Here's how the part is built. I have some questions about the finished solid (model axes, mm). A direction names the side the tool comes from. Coordinates: 2 decimals unless noted, no trailing zeros. Write each loop counter-clockwise with the first axis right and the second up, starting at its lowest first coordinate (ties: lowest second). Pieces come first, ordered by that corner, then holes. Notation, with made-up numbers: (26.5, 31.5) -> (53.5, 31.5) arc R26 cw to (53.5, 48.5) -> close; hole circle Ø11 at (78, 75). An arc over 180 degrees is marked (long way). Use CSV: the item, a comma, the result in double quotes. Start each with the question number.
```python
from build123d import *

# Parameters (mm, degrees)
SKETCH1_R           = 6.35
SKETCH1_R_2         = 1.8288
BOSS_EXTRUDE1_DEPTH = 6.35
SKETCH2_W           = 26.667
SKETCH2_H           = 26.667
BOSS_EXTRUDE2_DEPTH = 6.35


with BuildPart() as part:
    # Sketch1 → Boss-Extrude1 (new body)
    with BuildSketch(Plane(origin=(0, 0, 0), x_dir=(1, 0, 0), z_dir=(0, 1, 0))):
        Polygon((-35.064474094, 47.36223941), (-35.064474094, 7.36323941), (-35.064474094, -30.73676059), (3.035525906, -30.73676059), (3.035525906, 7.36323941), (3.035525906, 47.36223941), align=None)
        with Locations(Location((-16.014474094, -11.68676059, 0), (0, 0, 270))):
            Circle(SKETCH1_R, mode=Mode.SUBTRACT)
        with Locations(Location((-16.014474094, -21.46576059, 0), (0, 0, 270))):
            Circle(SKETCH1_R_2, mode=Mode.SUBTRACT)
        with Locations(Location((-22.929271308, -18.601557803, 0), (0, 0, 270))):
            Circle(SKETCH1_R_2, mode=Mode.SUBTRACT)
        with Locations(Location((-25.793474094, -11.68676059, 0), (0, 0, 270))):
            Circle(SKETCH1_R_2, mode=Mode.SUBTRACT)
        with Locations(Location((-22.929271308, -4.771963377, 0), (0, 0, 270))):
            Circle(SKETCH1_R_2, mode=Mode.SUBTRACT)
        with Locations(Location((-16.014474094, -1.90776059, 0), (0, 0, 270))):
            Circle(SKETCH1_R_2, mode=Mode.SUBTRACT)
        with Locations(Location((-9.099676881, -4.771963377, 0), (0, 0, 270))):
            Circle(SKETCH1_R_2, mode=Mode.SUBTRACT)
        with Locations(Location((-6.235474094, -11.68676059, 0), (0, 0, 270))):
            Circle(SKETCH1_R_2, mode=Mode.SUBTRACT)
        with Locations(Location((-9.099676881, -18.601557803, 0), (0, 0, 270))):
            Circle(SKETCH1_R_2, mode=Mode.SUBTRACT)
    extrude(amount=BOSS_EXTRUDE1_DEPTH)

    # Sketch2 → Boss-Extrude2 (add)
    with BuildSketch(Plane(origin=(0, 6.35, 0), x_dir=(1, 0, 0), z_dir=(0, 1, 0))):
        with Locations((-16.014474094, 47.36223941)):
            Rectangle(SKETCH2_W, SKETCH2_H)
    extrude(amount=-BOSS_EXTRUDE2_DEPTH)


solid = part.part
```
Item 1: Which directions (+Z, -Z, +X, -X, +Y, -Y) give clear straight access to the entire face, cutting with the end or side of a thin tool? Please do faces 5 (the cylindrical face through (-27.58, 3.13, 11.29)), 6 (the flat face through (0, 3, -47.362)), 7 (the flat face through (-29.348, 3, -54)).
Item 2: Thinking about a two-plate mould opening in Z: for faces 1 (the cylindrical face through (-21.116, 3.131, 4.534)), 2 (the flat face through (-16, 0, -16)), 3 (the flat face through (-32, 3, -47.362)), 4 (the cylindrical face through (-15.47, 3.13, 23.21)), which applies, +Z half, -Z half, draft (parallel to the pull), parting line (faces both ways), or undercut?
Item 3: I'm going to push flat-ended pins straight in: pin 1 (3 mm diameter, centred on x = -31.5, y = 2, fed in from -Z); pin 2 (3.5 mm diameter, centred on x = -9.1, z = 4.77, fed in from +Y); pin 3 (2 mm diameter, centred on y = 5, z = -49, fed in from +X); pin 4 (1.9 mm diameter, centred on y = 4.5, z = -57, fed in from -X). Where does each tip first touch, or does it pass through?
Item 4: If I drill on line 1 along Z through (x, y) = (-7.5, 4); line 2 along Z through (x, y) = (-31.5, 3.25); line 3 along X through (y, z) = (3, -47.5), over which ranges is the centre line in solid material (lowest first)?
Item 5: I want a section at C-C on x = 0.5. Please give me the cut outline in (y, z), then the cut area to 3 significant figures.
Item 6: I want a section at D-D on z = -49.5. Please give me the cut outline in (x, y), then the cut area to 3 significant figures.
Item 7: I want a section at B-B on y = 1.5. Count the separate pieces of the cut face and the enclosed holes in it, then the cut area to 3 significant figures.
Item 8: I want a section at A-A on z = 21.5. Please give me the cut outline in (x, y).
Geometry says:
1,face 5,"+Y, -Y"
1,face 6,"-Z, +X, +Y, -Y"
1,face 7,"-Z, -X, +Y, -Y"
2,face 1,"undercut"
2,face 2,"draft"
2,face 3,"-Z half"
2,face 4,"undercut"
3,pin 1,"z = -47.36"
3,pin 2,"through"
3,pin 3,"x = -2.68"
3,pin 4,"x = -29.35"
4,line 1,"-60.7 to 3.89, 5.66 to 10.37, 13.01 to 17.72, 19.49 to 30.74"
4,line 2,"-47.36 to 30.74"
4,line 3,"-29.35 to -2.68"
5,outline,"(0, -47.36) -> (6.35, -47.36) -> (6.35, 30.74) -> (0, 30.74) -> close"
5,area,"496 mm2"
6,outline,"(-29.35, 0) -> (-2.68, 0) -> (-2.68, 6.35) -> (-29.35, 6.35) -> close"
6,area,"169 mm2"
7,separate pieces,"1"
7,enclosed holes,"9"
7,area,"3,120 mm2"
8,outline,"(-35.06, 0) -> (-17.84, 0) -> (-17.84, 6.35) -> (-35.06, 6.35) -> close; (-14.19, 0) -> (3.04, 0) -> (3.04, 6.35) -> (-14.19, 6.35) -> close"
